Check sheet for the drawn part. Datum: minimum x, y, z corner. Units: mm. Round coordinates to 2 decimals unless told otherwise and drop trailing zeros. Order: outer loops, then holes, each group sorted by start corner. A loop starts at its lowest first (then second) coordinate and runs counter-clockwise, first axis right, second up. Notation, with made-up numbers: M -0.75,-18.5 L 21.25,-18.5 A7 cw 21.25,-10.5 Z; hole C -33,-38 d8. An arc over 180 degrees is marked long. Answer as a JSON object with one key per item and string values. Group by question number.
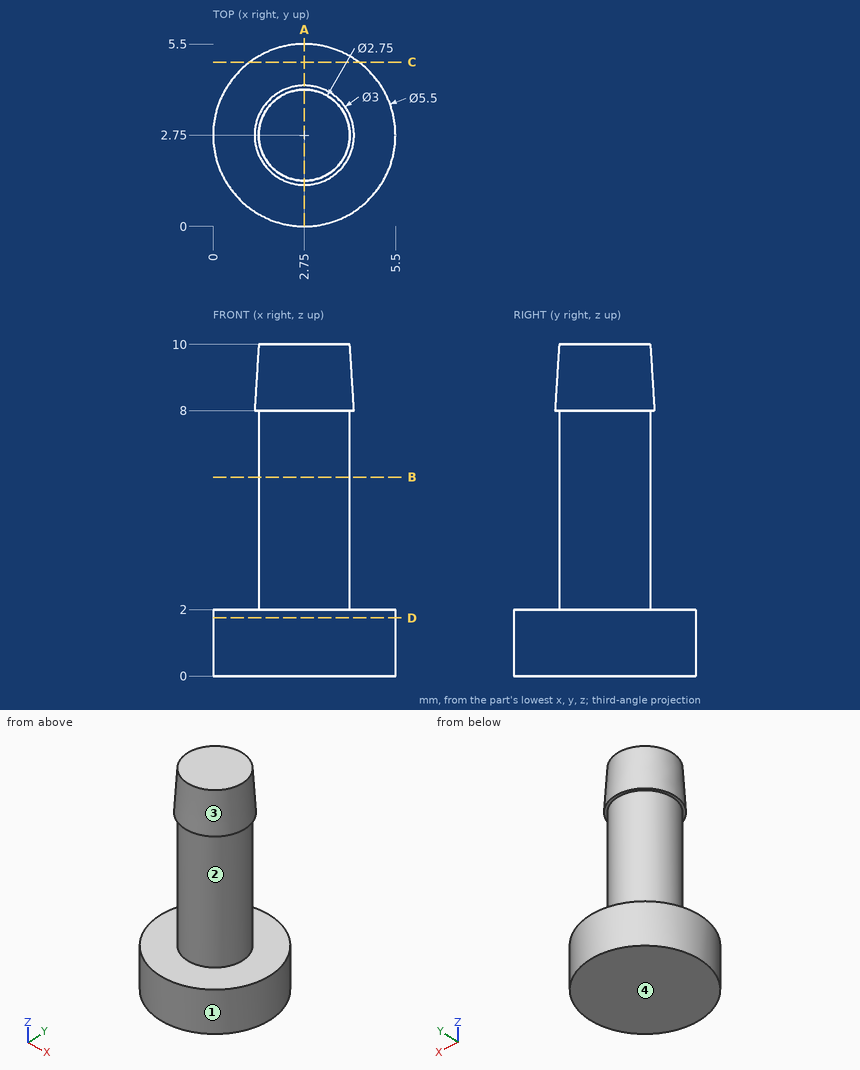
1) Sectioned sample at B-B (z = 6). Record the boundary of the cut face in (x, y) (3 decimals), then the cut area to 3 significant figures.
2) Release check for a two-part mould opening along Z. For the marked faces 1, 2, 3 and 4 record: +Z half, -Z half, draft (parallel to the pull), parting line (faces both ways), or undercut.
3) Go/stop test with flat-tipped pins: P1, Ø3, axis at x = 4, y = 4, coming from the +Z side; P2, Ø3, axis at y = 2.5, z = 7, coming from the -X side; P3, Ø3, axis at x = 4.5, z = 2, coming from the -Y side; P4, Ø2, axis at y = 1.5, z = 3.5, coming from the +X side. Record where each tip stops, or that it passes through.
4) Thickness scan on line 1 along Z through (x, y) = (0.55, 1.7); line 2 along Y through (x, z) = (2.5, 9); line 3 along X through (y, z) = (2.45, 3.5). Record the ranges inside material, lowest first. Write a range as [from, to].
5) Sectioned sample at C-C (y = 4.95). Record the boundary of the cut face in (x, z), then the cut area to 3 significant figures.
6) Sectioned sample at D-D (z = 1.75). Record the boundary of the cut face in (x, y).
7) Sectioned sample at A-A (x = 2.75). Record the boundary of the cut face in (y, z) (3 decimals), then the cut area to 4 significant figures.
Final values:
{
 "1": {"outline": "C 2.75,2.75 d2.75", "area": "5.94 mm^2"},
 "2": {"face 1": "draft", "face 2": "undercut", "face 3": "+Z half", "face 4": "-Z half"},
 "3": {"P1": "stops at z = 10", "P2": "stops at x = 1.25", "P3": "stops at y = 0.01", "P4": "stops at x = 4.1"},
 "4": {"line 1": "z = [0, 2]", "line 2": "y = [1.33, 4.17]", "line 3": "x = [1.41, 4.09]"},
 "5": {"outline": "M 1.1,0 L 4.4,0 L 4.4,2 L 1.1,2 Z", "area": "6.60 mm^2"},
 "6": {"outline": "C 2.75,2.75 d5.5"},
 "7": {"outline": "M 0,0 L 5.5,0 L 5.5,2 L 4.125,2 L 4.125,8 L 4.25,8 L 4.125,10 L 1.375,10 L 1.25,8 L 1.375,8 L 1.375,2 L 0,2 Z", "area": "33.25 mm^2"}
}
